Job drawing, mm, ordinate dimensions from the low corner. One solid piece. Coordinates: 2 decimals unless noted, no trailing zeros. Order: outer loops, then holes, each group sorted by start corner. A loop starts at its lowest first (then second) coordinate and runs counter-clockwise, first axis right, second up. Notation, with made-up numbers: M 41,11 L 80,11 A12 ccw 80,33 Z; hole C -18,-39 d9. An arc over 180 degrees is marked long. Write item = value, one per line. Start each with the question number.
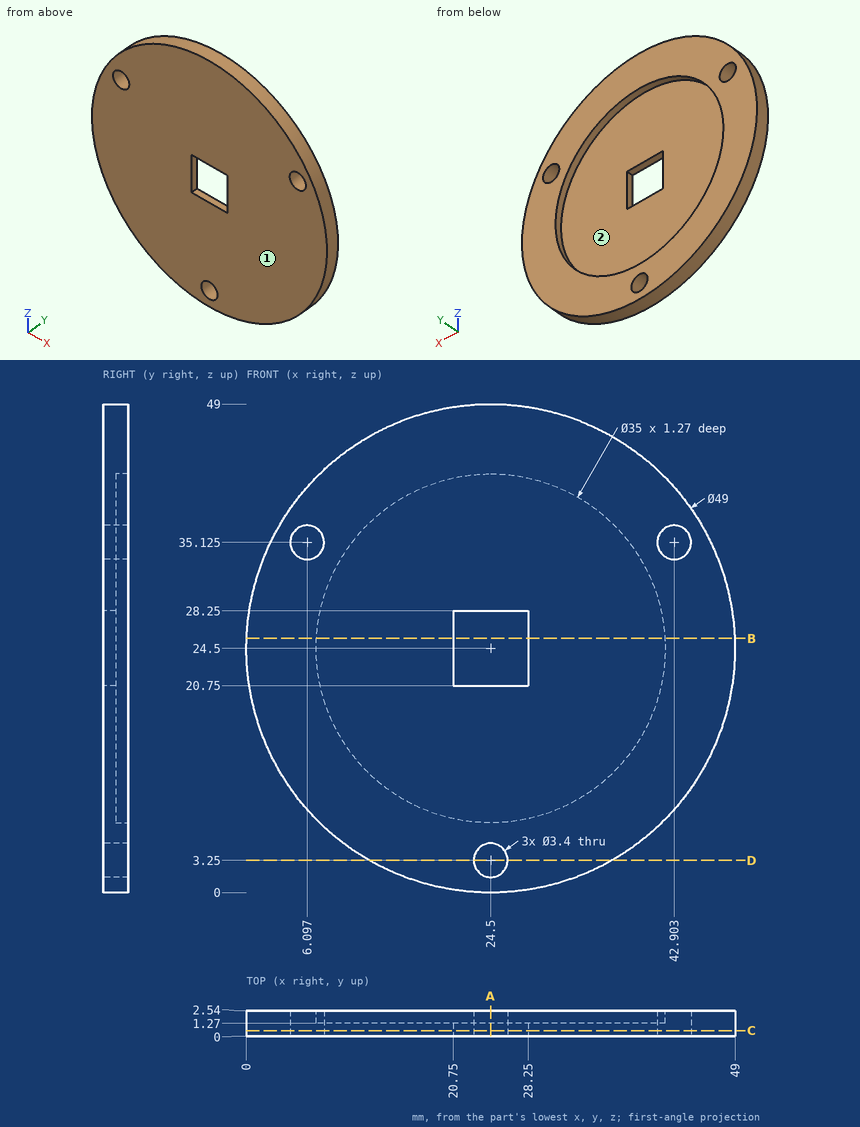
Item 1: Cut at B-B, the plane z = 25.5. Write the cut outline in (x, y).
Item 2: Cut at C-C, the plane y = 0.55. Write the cut outline in (x, z) (3 decimals).
Item 3: Flat gauge pins, fed straight in: pin 1 (1 mm diameter, centred on y = 0.5, z = 25, fed in from -X); pin 2 (5 mm diameter, centred on x = 5.5, z = 35, fed in from +Y); pin 3 (1.4 mm diameter, centred on x = 23.5, y = 0.5, fed in from -Z); pin 4 (17.5 mm diameter, centred on x = 26, z = 18, fed in from +Y). Where does each tip first touch, or does it go through?
Item 4: Cut at A-A, the plane x = 24.5. Write the cut outline in (y, z).
Item 5: Wall check: line 1 along X through (y, z) = (1.65, 24.5); line 2 along Z through (x, y) = (25.5, 2.4); line 3 along X through (y, z) = (2.2, 36.5). Give the ranges that are in metal, low to high. Write a range as [from, to].
Item 6: Pull direction Z, two halves, no side cores. Call the marked faces 1 and 2: pulls with the +Z half, pulls with the -Z half, needs draft (parallel to the pull), parting line crosses it, or undercut.
Item 7: Cut at D-D, the plane z = 3.25. Write the cut outline in (x, y), and give its area (3 significant figures).
Filled sheet:
q1.outline = M 0.02,0 L 20.75,0 L 20.75,1.27 L 7.03,1.27 L 7.03,2.54 L 0.02,2.54 Z; M 28.25,0 L 48.98,0 L 48.98,2.54 L 41.97,2.54 L 41.97,1.27 L 28.25,1.27 Z
q2.outline = C 24.5,24.5 d49; hole C 6.097,35.125 d3.4; hole M 20.75,20.75 L 28.25,20.75 L 28.25,28.25 L 20.75,28.25 Z; hole C 24.5,3.25 d3.4; hole C 42.903,35.125 d3.4
q3.pin_1 = 0
q3.pin_2 = 2.54
q3.pin_3 = 0
q3.pin_4 = 1.27
q4.outline = M 0,0 L 2.54,0 L 2.54,1.55 L 0,1.55 Z; M 0,4.95 L 2.54,4.95 L 2.54,7 L 1.27,7 L 1.27,20.75 L 0,20.75 Z; M 0,28.25 L 1.27,28.25 L 1.27,42 L 2.54,42 L 2.54,49 L 0,49 Z
q5.line_1 = [0, 7], [42, 49]
q5.line_2 = [0.02, 1.88], [4.62, 7.03], [41.97, 48.98]
q5.line_3 = [3.14, 5.1], [7.1, 11.76], [37.24, 41.9], [43.9, 45.86]
q6.face_1 = needs draft
q6.face_2 = undercut
q7.outline = M 12.31,0 L 22.8,0 L 22.8,2.54 L 12.31,2.54 Z; M 26.2,0 L 36.69,0 L 36.69,2.54 L 26.2,2.54 Z
q7.area = 53.3 mm2
